from build123d import *

# Parameters (mm, degrees)
SKETCH_W    = 80
SKETCH_H    = 120
SKETCH_R    = 9.5
SKETCH_R_2  = 3
PAD_DEPTH   = 10
FILLET_R    = 1
FILLET001_R = 10


with BuildPart() as part:
    # Sketch → Pad (new body)
    with BuildSketch(Plane.XY):
        with Locations((15, -15)):
            Rectangle(SKETCH_W, SKETCH_H)
        with Locations((0, -30)):
            Circle(SKETCH_R, mode=Mode.SUBTRACT)
        with Locations((-10, -52)):
            Circle(SKETCH_R_2, mode=Mode.SUBTRACT)
        with Locations((40, -52)):
            Circle(SKETCH_R_2, mode=Mode.SUBTRACT)
        with Locations((40, 22)):
            Circle(SKETCH_R_2, mode=Mode.SUBTRACT)
        with Locations((-10, 22)):
            Circle(SKETCH_R_2, mode=Mode.SUBTRACT)
        with BuildLine():
            ThreePointArc((-5, -6.244998), (8, 0), (-5, 6.244998))
            Line((-5, 9), (-5, 6.244998))
            Line((-8.125, 9), (-5, 9))
            Line((-8.125, -9), (-8.125, 9))
            Line((-5, -9), (-8.125, -9))
            Line((-5, -6.244998), (-5, -9))
        make_face(mode=Mode.SUBTRACT)
    extrude(amount=PAD_DEPTH)

    # Fillet
    fillet_edges = [part.edges().sort_by_distance(p)[0] for p in [
        (55, -75, 5),
        (55, 45, 5),
    ]]
    fillet(fillet_edges, radius=FILLET_R)

    # Fillet001
    fillet001_edges = [part.edges().sort_by_distance(p)[0] for p in [
        (-25, -75, 5),
        (-25, 45, 5),
    ]]
    fillet(fillet001_edges, radius=FILLET001_R)


solid = part.part
Build history of the part. All positions in model axes, mm. A direction names the side the tool comes from. Round coordinates to 2 decimals unless told otherwise and drop trailing zeros. Loops run counter-clockwise (first coordinate to the right, second up) from the corner with the lowest first, then second, coordinate; pieces in that order, holes last. Notation, with made-up numbers: (73, 79) -> (132, 79) arc R25 ccw to (132, 115) -> close; hole circle Ø6 at (10, 54.25). An arc over 180 degrees is marked (long way). Use CSV: the item, a comma, the result in double quotes. Start each with the question number.
Q1. Saw through at B-B on x = 0. Give the cut face in (y, z), and give its area (3 significant figures).
Q2. Which spindle directions (+Z, -Z, +X, -X, +Y, -Y) get a long thin tool onto all of the face, cutting with end or side? Do faces 1 (the face through (-8.125, 0, 5)), 2 (the face through (19, 45, 5)). Say none if no direction does.
Q3. Flat gauge pin, fed straight in: pin 1 Ø2 at (x, y) = (-16.5, -50) entering from -Z. Where does the tip first touch, or does it go through?
Q4. Saw through at A-A on y = -30. Give the cut face in (x, z).
Q5. Saw through at C-C on y = 22. Give the cut face in (x, z).
Q6. Drill centre lines: L1, parallel to Y at x = 0, z = 3; L2, parallel to Y at x = 40, z = 7; L3, parallel to Y at x = -7.5, z = 6.5. Where is each one in solid material? Low to high.
Q7. Mould opens along X. For faces 3 (the face through (55, -16, 5)), 4 (the face through (14, -14, 10)), 5 (the face through (-7, -9, 5)) say: +X half, -X half, draft (parallel to the pull), parting line (faces both ways), or undercut.
Solutions:
1,outline,"(-75, 0) -> (-39.5, 0) -> (-39.5, 10) -> (-75, 10) -> close; (-20.5, 0) -> (-8, 0) -> (-8, 10) -> (-20.5, 10) -> close; (8, 0) -> (45, 0) -> (45, 10) -> (8, 10) -> close"
1,area,"850 mm^2"
2,face 1,"+Z, -Z"
2,face 2,"+Z, -Z, +X, -X, +Y"
3,pin 1,"stops at z = 0"
4,outline,"(-25, 0) -> (-9.5, 0) -> (-9.5, 10) -> (-25, 10) -> close; (9.5, 0) -> (55, 0) -> (55, 10) -> (9.5, 10) -> close"
5,outline,"(-25, 0) -> (-13, 0) -> (-13, 10) -> (-25, 10) -> close; (-7, 0) -> (37, 0) -> (37, 10) -> (-7, 10) -> close; (43, 0) -> (55, 0) -> (55, 10) -> (43, 10) -> close"
6,L1,"y = -75 to -39.5, -20.5 to -8, 8 to 45"
6,L2,"y = -75 to -55, -49 to 19, 25 to 45"
6,L3,"y = -75 to -53.66, -50.34 to -35.83, -24.17 to -9, 9 to 20.34, 23.66 to 45"
7,face 3,"+X half"
7,face 4,"draft"
7,face 5,"undercut"
